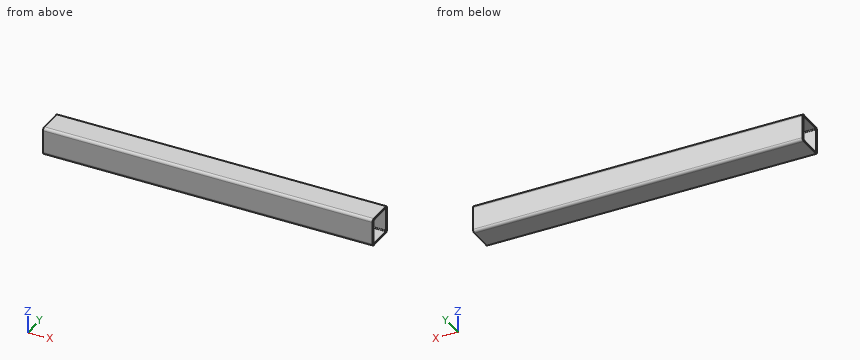
```python
from build123d import *

# Parameters (mm, degrees)
F1_DEPTH = 1200.15


with BuildPart() as f1:
    # F0 (on Right) → F1 (new body)
    with BuildSketch(Plane.YZ):
        with BuildLine():
            ThreePointArc((0, 9.525), (2.789808, 2.789808), (9.525, 0))
            Line((9.525, 0), (92.075, 0))
            ThreePointArc((92.075, 0), (98.810192, 2.789808), (101.6, 9.525))
            Line((101.6, 9.525), (101.6, 92.075))
            ThreePointArc((101.6, 92.075), (98.810192, 98.810192), (92.075, 101.6))
            Line((92.075, 101.6), (9.525, 101.6))
            ThreePointArc((9.525, 101.6), (2.789808, 98.810192), (0, 92.075))
            Line((0, 92.075), (0, 9.525))
        make_face()
        with BuildLine():
            ThreePointArc((95.25, 9.525), (94.320064, 7.279936), (92.075, 6.35))
            Line((92.075, 6.35), (9.525, 6.35))
            ThreePointArc((9.525, 6.35), (7.279936, 7.279936), (6.35, 9.525))
            Line((6.35, 9.525), (6.35, 92.075))
            ThreePointArc((6.35, 92.075), (7.279936, 94.320064), (9.525, 95.25))
            Line((9.525, 95.25), (92.075, 95.25))
            ThreePointArc((92.075, 95.25), (94.320064, 94.320064), (95.25, 92.075))
            Line((95.25, 92.075), (95.25, 9.525))
        make_face(mode=Mode.SUBTRACT)
    extrude(amount=F1_DEPTH)


solid = f1.part
```
Here's how the part is built. I have some questions about the finished solid (model axes, mm). Coordinates: 2 decimals unless noted, no trailing zeros. Loops run counter-clockwise (first coordinate to the right, second up) from the corner with the lowest first, then second, coordinate; pieces in that order, holes last. Notation, with made-up numbers: (16, -8) - (22, -8) arc R10 ccw to (22, 3) - close; hole circle Ø10 at (18, -19). An arc over 180 degrees is marked (long way). Answer as CSV lines item,"result".
Q1. If I drill on L1, parallel to Z at x = 186, y = 87.5, over which ranges is the centre line in solid material (lowest first)? Write a range as [from, to].
Response:
L1,"[0, 6.35], [95.25, 101.6]"
Q2. If we section it at C-C, the plane x = 497.5: Write out the boundary of the cut face in (y, z) (3 decimals).
Response:
outline,"(0, 9.525) arc R9.525 ccw to (9.525, 0) - (92.075, 0) arc R9.525 ccw to (101.6, 9.525) - (101.6, 92.075) arc R9.525 ccw to (92.075, 101.6) - (9.525, 101.6) arc R9.525 ccw to (0, 92.075) - close; hole (6.35, 9.525) arc R3.175 ccw to (9.525, 6.35) - (92.075, 6.35) arc R3.175 ccw to (95.25, 9.525) - (95.25, 92.075) arc R3.175 ccw to (92.075, 95.25) - (9.525, 95.25) arc R3.175 ccw to (6.35, 92.075) - close"
Q3. If we section it at A-A, the plane z = 48.5: Write out the boundary of the cut face in (x, y).
Response:
outline,"(0, 0) - (1200.15, 0) - (1200.15, 6.35) - (0, 6.35) - close; (0, 95.25) - (1200.15, 95.25) - (1200.15, 101.6) - (0, 101.6) - close"
